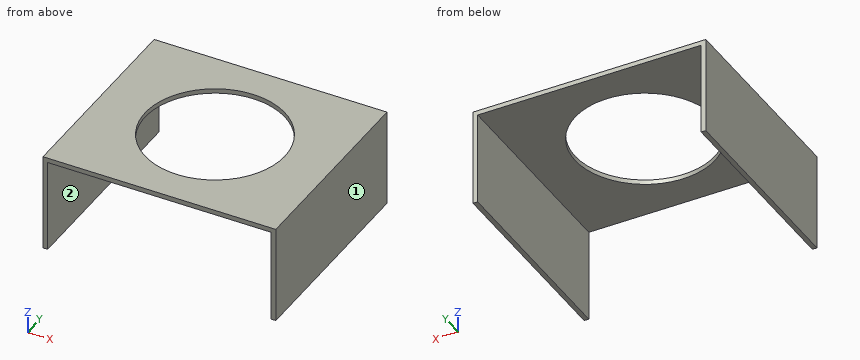
from build123d import *

# Parameters (mm, degrees)
SKETCH1_W           = 50.000000596
SKETCH1_H           = 43.88833532
BOSS_EXTRUDE1_DEPTH = 1
SKETCH2_W           = 1
SKETCH2_H           = 43.88833532
BOSS_EXTRUDE3_DEPTH = 20
SKETCH3_R           = 15
CUT_EXTRUDE1_DEPTH  = 40.338867665


with BuildPart() as part:
    # Sketch1 → Boss-Extrude1 (new body)
    with BuildSketch(Plane.XY):
        Rectangle(SKETCH1_W, SKETCH1_H)
    extrude(amount=BOSS_EXTRUDE1_DEPTH)

    # Sketch2 → Boss-Extrude3 (add)
    with BuildSketch(Plane(origin=(0, 0, 0), x_dir=(-1, 0, 0), z_dir=(0, 0, -1))):
        Polygon((25.000000298, 21.94416766), (24.000000298, 21.94416766), (24.000000298, -21.94416766), (25.000000298, -21.94416766), (25.000000298, 21.001254621), align=None)
        with Locations((-24.500000298, 0)):
            Rectangle(SKETCH2_W, SKETCH2_H)
    extrude(amount=BOSS_EXTRUDE3_DEPTH)

    # Sketch3 → Cut-Extrude1 (cut, through all)
    with BuildSketch(Plane.XY.offset(1)):
        Circle(SKETCH3_R)
    extrude(amount=-CUT_EXTRUDE1_DEPTH, mode=Mode.SUBTRACT)


solid = part.part
Could you check a few things on this model? Use its own coordinates, in mm. Face numbers are marked on the shaded views. A direction names the side the tool comes from. Give positions to 0.01 mm unless a question says otherwise; leave off trailing zeros. Order: outer loops, then holes, each group sorted by start corner. A loop starts at its lowest first (then second) coordinate and runs counter-clockwise, first axis right, second up. Notation, with made-up numbers: (62.25, -12.5) - (73.25, -12.5) arc R29 cw to (73.25, 16.5) - close; hole circle Ø1 at (35, -5). An arc over 180 degrees is marked (long way). One line per item, written item: value. Start each with the question number.
1. Imagine slicing it at C-C on y = 0. List the corners of the cut face in (x, z) for me.
2. Imagine slicing it at D-D on y = 11. List the corners of the cut face in (x, z) for me.
3. Imagine slicing it at A-A on z = -18.5. List the corners of the cut face in (x, y) for me, plus the area to 3 significant figures.
4. If I drill on probe 1 along Y at (x, z) = (0, 0.8); probe 2 along X at (y, z) = (-17, -4.5); probe 3 along Z at (x, y) = (20, 15.5), over which ranges is the centre line in solid material (lowest first)?
5. Imagine slicing it at B-B on x = 0. List the corners of the cut face in (y, z) for me.
6. For P1, Ø13, axis at x = 8, y = 6, coming from the -Z side, with a flat end and sliding along its axis, tell me the tip position at first contact or that it passes through.
7. For the marked faces 1 and 2, which set-ups out of +Z, -Z, +X, -X, +Y, -Y let a thin tool reach every point of the face, with its end or its side?
Values:
1. outline: (-25, -20) - (-24, -20) - (-24, 0) - (-15, 0) - (-15, 1) - (-25, 1) - close; (15, 0) - (24, 0) - (24, -20) - (25, -20) - (25, 1) - (15, 1) - close
2. outline: (-25, -20) - (-24, -20) - (-24, 0) - (-10.2, 0) - (-10.2, 1) - (-25, 1) - close; (10.2, 0) - (24, 0) - (24, -20) - (25, -20) - (25, 1) - (10.2, 1) - close
3. outline: (-25, -21.94) - (-24, -21.94) - (-24, 21.94) - (-25, 21.94) - close; (24, -21.94) - (25, -21.94) - (25, 21.94) - (24, 21.94) - close
3. area: 87.8 mm²
4. probe 1: -21.94 to -15, 15 to 21.94
4. probe 2: -25 to -24, 24 to 25
4. probe 3: 0 to 1
5. outline: (-21.94, 0) - (-15, 0) - (-15, 1) - (-21.94, 1) - close; (15, 0) - (21.94, 0) - (21.94, 1) - (15, 1) - close
6. P1: z = 0
7. face 1: +Z, -Z, +X, +Y, -Y
7. face 2: -Z, +Y, -Y
